Solid Edge part; units mm, degrees
sketch "Sketch1" plane through (0, 0, 0) normal (0, -1, 0) x (1, 0, 0)
  line L0 (16, 20) -> (-44, 20)
  line L1 (-44, 20) -> (-44, -20)
  line L2 (-44, -20) -> (16, -20)
  line L3 (16, -20) -> (16, 20)
  dimension "D1" = 16
  dimension "D2" = 16
extrude "Protrusion1" add sketch "Sketch1" against normal blind 24.5
sketch "Sketch2" plane through (-14, 0, 0) normal (0, -1, 0) x (0, 0, -1)
  circle A0 centre (0, 14) radius 11.5
extrude "Cutout1" cut sketch "Sketch2" against normal through all
sketch "Sketch3" plane through (-14, 24.5, 0) normal (0, 1, 0) x (0, 0, 1)
  line L0 (-16, -24.5) -> (16, -24.5)
  line L1 (16, -24.5) -> (16, 25.5)
  line L2 (16, 25.5) -> (-16, 25.5)
  line L3 (-16, 25.5) -> (-16, -24.5)
  dimension "D1" = 16
  dimension "D2" = 16
extrude "VaciadoExtruido_2" cut sketch "Sketch3" against normal blind 10
sketch "Sketch4" plane through (-13.5, 14.5, 0) normal (0, 1, 0) x (0, 0, 1)
  line L0 (-10.5, -19.5) -> (10.5, -19.5)
  line L1 (10.5, -19.5) -> (10.5, 13.5)
  line L2 (10.5, 13.5) -> (-10.5, 13.5)
  line L3 (-10.5, 13.5) -> (-10.5, -19.5)
  dimension "D1" = 10.5
  dimension "D2" = 10.5
extrude "VaciadoExtruido_3" cut sketch "Sketch4" against normal blind 3
sketch "Sketch5" plane through (-14, 0, 15) normal (0, -1, 0) x (-1, 0, 0)
  circle A0 centre (-7.5, 28.5) radius 1.3
  circle A1 centre (8.5, 28.5) radius 1.1
  circle A2 centre (16.5, 28.5) radius 1.1
  circle A3 centre (-7.5, 1.5) radius 1.3
  circle A4 centre (0.5, 1.5) radius 1.3
  circle A5 centre (8.5, 1.5) radius 1.3
  circle A6 centre (16.5, 1.5) radius 1.3
  circle A7 centre (22, 23) radius 1.3
  circle A8 centre (22, 7) radius 1.3
  circle A9 centre (0.5, 28.5) radius 1.3
extrude "Cutout2" cut sketch "Sketch5" against normal up to vertex (14.5 mm away)
sketch "Sketch6" plane through (-14, 0, 15) normal (0, -1, 0) x (-1, 0, 0)
  circle A0 centre (-7.5, 1.5) radius 3.25
  circle A1 centre (0.5, 1.5) radius 3.25
  circle A2 centre (8.5, 1.5) radius 3.25
  circle A3 centre (16.5, 1.5) radius 3.25
  circle A4 centre (22, 7) radius 3.25
  circle A5 centre (22, 23) radius 3.25
  circle A6 centre (16.5, 28.5) radius 3.25
  circle A7 centre (0.5, 28.5) radius 3.25
  circle A8 centre (8.5, 28.5) radius 3.25
  circle A9 centre (-7.5, 28.5) radius 3.25
extrude "Cutout3" cut sketch "Sketch6" against normal blind 12
sketch "Sketch7" plane through (-14, 0, 0) normal (0, -1, 0) x (-1, 0, 0)
  line L0 (30, 20) -> (-30, 20)
  line L1 (-30, 20) -> (-30, -20)
  line L2 (-30, -20) -> (30, -20)
  line L3 (30, -20) -> (30, 20)
extrude "VaciadoExtruido_10" cut sketch "Sketch7" against normal blind 10.5
sketch "Sketch8" plane through (-14, 24.5, 0) normal (0, 1, 0) x (1, 0, 0)
  line L0 (-30, 20) -> (30, 20)
  line L1 (30, 20) -> (30, -20)
  line L2 (30, -20) -> (-30, -20)
  line L3 (-30, -20) -> (-30, 20)
  line L4 (-24.5, 16) -> (-24.5, -16)
  line L5 (-24.5, -16) -> (25.5, -16)
  line L6 (25.5, -16) -> (25.5, 16)
  line L7 (25.5, 16) -> (-24.5, 16)
extrude "ProtrusiónExtruida_7" add sketch "Sketch8" along normal blind 36
sketch "Sketch9" plane through (16, 35.5, 0) normal (1, 0, 0) x (0, 1, 0)
  line L0 (25, -20) -> (25, 20)
  line L1 (25, 20) -> (15, 20)
  line L2 (15, 20) -> (15, -20)
  line L3 (25, -20) -> (15, -20)
  dimension "D1" = 25
extrude "ProtrusiónExtruida_8" add sketch "Sketch9" along normal blind 17
sketch "Sketch10" plane through (-5.5, 35.5, 20) normal (0, 0, 1) x (-1, 0, 0)
  line L0 (-36.5, -25) -> (-36.5, -23)
  line L1 (-36.5, -23) -> (-21.5, -23)
  line L2 (-21.5, -23) -> (-21.5, -25)
  dimension "D1" = 36.5
extrude "Cutout4" cut sketch "Sketch10" against normal up to next material side at (30.95, 59.5, 20)
sketch "Sketch11" plane through (-5.5, 35.5, 20) normal (0, 0, 1) x (-1, 0, 0)
  line L0 (38.5, 25) -> (-21.5, 25)
  line L1 (-21.5, -15) -> (-21.5, 25)
  line L2 (-38.5, -15) -> (-21.5, -15)
  line L3 (-38.5, -15) -> (-38.5, -25)
  line L4 (-38.5, -25) -> (-36.5, -25)
  line L5 (-36.5, -25) -> (-36.5, -23)
  line L6 (-36.5, -23) -> (-21.5, -23)
  line L7 (-21.5, -25) -> (-21.5, -23)
  line L8 (38.5, -25) -> (-21.5, -25)
  line L9 (38.5, -25) -> (38.5, 25)
extrude "Protrusion2" add sketch "Sketch11" along normal blind 5
sketch "Sketch12" plane through (-5.5, 35.5, -20) normal (0, 0, -1) x (-1, 0, 0)
  line L0 (-38.5, 25) -> (-36.5, 25)
  line L1 (-36.5, 25) -> (-36.5, 23)
  line L2 (-36.5, 23) -> (-21.5, 23)
  line L3 (-21.5, 23) -> (-21.5, 25)
  line L4 (-21.5, 25) -> (38.5, 25)
  line L5 (38.5, 25) -> (38.5, -25)
  line L6 (38.5, -25) -> (-21.5, -25)
  line L7 (-21.5, -25) -> (-21.5, 15)
  line L8 (-21.5, 15) -> (-38.5, 15)
  line L9 (-38.5, 15) -> (-38.5, 25)
extrude "ProtrusiónExtruida_10" add sketch "Sketch12" along normal blind 5
hole "Agujero_8" at (23.5, 58.5, 15) direction (0, -1, 0) diameter 6.5 end up to next
hole "Hole1" at (23.5, 58.5, 0) direction (0, -1, 0) diameter 6.5 end up to next
hole "Hole2" at (23.5, 58.5, -15) direction (0, -1, 0) diameter 6.5 end up to next
Design review of the part built by this model. Coordinates are the model's own, in mm. A direction names the side the tool comes from. Coordinates: 2 decimals unless noted, no trailing zeros. Write each loop counter-clockwise with the first axis right and the second up, starting at its lowest first coordinate (ties: lowest second). Pieces come first, ordered by that corner, then holes. Notation, with made-up numbers: (-29.75, 87) - (-11.75, 87) arc R11 cw to (-11.75, 98) - close; hole circle Ø2 at (4, 26). An arc over 180 degrees is marked (long way). One line per item, written item: value.
1) Add section A-A (x = 0). State the section outline as (y, z) points.
Answer sheet:
outline: (10.5, -25) - (60.5, -25) - (60.5, -16) - (14.5, -16) - (14.5, -11.5) - (10.5, -11.5) - close; (10.5, 11.5) - (14.5, 11.5) - (14.5, 16) - (60.5, 16) - (60.5, 25) - (10.5, 25) - close
2) To check wall thickness, follow probe 1 along Z at (x, y) = (-36, 11); probe 2 along Z at (x, y) = (-22.5, 11); probe 3 along X at (y, z) = (51, -9). State the ranges of each line that lie inside material, in increasing order.
Answer sheet:
probe 1: z = -25 to -11.25, -4.75 to 4.75, 11.25 to 25
probe 2: z = -25 to -16.75, -10.25 to 10.25, 16.75 to 25
probe 3: x = -44 to -38.5, 11.5 to 33
3) Insertion check: pin 1 (3 mm diameter, centred on x = -21, z = 13, fed in from -Y); pin 2 (4 mm diameter, centred on x = -22.5, z = 13.5, fed in from +Y); pin 3 (12 mm diameter, centred on y = 40.5, z = -1.5, fed in from +X); pin 4 (5 mm diameter, centred on x = 23.5, z = -15, fed in from -Y). Each pin has a flat end and moves straight along its axis. Give the tip position at first contact, or say it passes through.
Answer sheet:
pin 1: stops at y = 12
pin 2: stops at y = 14.5
pin 3: stops at x = 16
pin 4: passes through
4) Add section C-C (x = -30.5). State the section outline as (y, z) points, plus the area to 3 significant figures.
Answer sheet:
outline: (10.5, -25) - (60.5, -25) - (60.5, -16) - (14.5, -16) - (14.5, -14.6) - (12, -14.6) - (12, -16.75) - (10.5, -16.75) - close; (10.5, -10.25) - (11.5, -10.25) - (11.5, 10.25) - (10.5, 10.25) - close; (10.5, 16.75) - (12, 16.75) - (12, 14.8) - (14.5, 14.8) - (14.5, 16) - (60.5, 16) - (60.5, 25) - (10.5, 25) - close; (12, -12.4) - (14.5, -12.4) - (14.5, -10.5) - (12, -10.5) - close; (12, 10.5) - (14.5, 10.5) - (14.5, 12.2) - (12, 12.2) - close
area: 934 mm2
5) Add section B-B (x = 23.5). State the section outline as (y, z) points, plus the area to 3 significant figures.
Answer sheet:
outline: (50.5, -25) - (58.5, -25) - (58.5, -18.25) - (50.5, -18.25) - close; (50.5, -11.75) - (58.5, -11.75) - (58.5, -3.25) - (50.5, -3.25) - close; (50.5, 3.25) - (58.5, 3.25) - (58.5, 11.75) - (50.5, 11.75) - close; (50.5, 18.25) - (58.5, 18.25) - (58.5, 25) - (50.5, 25) - close
area: 244 mm2
6) Add section D-D (z = 1.5). State the section outline as (x, y) points.
Answer sheet:
outline: (-44, 10.5) - (-11.4, 10.5) - (-11.4, 11.5) - (-33, 11.5) - (-33, 14.5) - (-38.5, 14.5) - (-38.5, 60.5) - (-44, 60.5) - close; (11.4, 10.5) - (16, 10.5) - (16, 50.5) - (20.62, 50.5) - (20.62, 58.5) - (16, 58.5) - (16, 60.5) - (11.5, 60.5) - (11.5, 14.5) - (11.4, 14.5) - close; (26.38, 50.5) - (33, 50.5) - (33, 60.5) - (31, 60.5) - (31, 58.5) - (26.38, 58.5) - close
7) For faces 1 (the face through (-39.1, 11.24, 7.02)), 2 (the face through (-22, 11.5, 0)), 3 (the face through (27, 58.5, 0)), list the 3-axis set-ups (+Z, -Z, +X, -X, +Y, -Y) from which the entire face can be reached by the end or side of a thin tool; tool diameter is ignored.
Answer sheet:
face 1: -Y
face 2: +Y
face 3: +Z, -Z, +Y
